from build123d import *

# Parameters (mm, degrees)
SKETCH1_R           = 1.5
SKETCH1_R_2         = 1
SKETCH1_W           = 2
SKETCH1_H           = 7
BOSS_EXTRUDE1_DEPTH = 5


with BuildPart() as part:
    # Sketch1 → Boss-Extrude1 (new body)
    with BuildSketch(Plane.XY):
        with BuildLine():
            Line((10.74521866, -60), (-20.072092256, -60))
            ThreePointArc((-20.072092256, -60), (-4.663436798, -26.922179377), (10.74521866, -60))
        make_face()
        with Locations((7.518690065, -56.019210774)):
            Circle(SKETCH1_R, mode=Mode.SUBTRACT)
        with Locations((-18.522064611, -53.115425948)):
            Circle(SKETCH1_R, mode=Mode.SUBTRACT)
        with Locations((-2.986935847, -32.015363278)):
            Circle(SKETCH1_R, mode=Mode.SUBTRACT)
        with Locations((1.346970842, -41.03959236)):
            Circle(SKETCH1_R_2, mode=Mode.SUBTRACT)
        with Locations((1.346970842, -53.06040764)):
            Circle(SKETCH1_R_2, mode=Mode.SUBTRACT)
        with Locations((-10.673844438, -53.06040764)):
            Circle(SKETCH1_R_2, mode=Mode.SUBTRACT)
        with Locations((-10.673844438, -41.03959236)):
            Circle(SKETCH1_R_2, mode=Mode.SUBTRACT)
        with Locations((-0.163436798, -47.05)):
            Rectangle(SKETCH1_W, SKETCH1_H, mode=Mode.SUBTRACT)
    extrude(amount=BOSS_EXTRUDE1_DEPTH)


solid = part.part
Build history of the part. All positions in model axes, mm. A direction names the side the tool comes from. Round coordinates to 2 decimals unless told otherwise and drop trailing zeros. Write each loop counter-clockwise with the first axis right and the second up, starting at its lowest first coordinate (ties: lowest second). Pieces come first, ordered by that corner, then holes. Notation, with made-up numbers: M -13,69.5 L 12,69.5 A23 cw 12,88.5 Z; hole C 75,56 d5. An arc over 180 degrees is marked long. Use CSV: the item, a comma, the result in double quotes.
1. Saw through at A-A (y = -47.05). Give the cut face in (x, z).
Reply:
outline,"M -24.79,0 L -1.16,0 L -1.16,5 L -24.79,5 Z; M 0.84,0 L 15.46,0 L 15.46,5 L 0.84,5 Z"
2. Wall check: probe 1 along X at (y, z) = (-53, 4.2); probe 2 along Y at (x, z) = (-11, 2.6); probe 3 along Y at (x, z) = (-10.5, 3.95). Give the ranges that are in metal, low to high. Write a range as from..to.
Reply:
probe 1,"x = -23.89..-20.02, -17.03..-11.67, -9.68..0.35, 2.35..14.56"
probe 2,"y = -60..-54.01, -52.12..-41.98, -40.09..-27.95"
probe 3,"y = -60..-54.05, -52.08..-42.02, -40.05..-27.79"
3. Saw through at D-D (x = 10). Give the cut face in (y, z), plus the area to 3 significant figures.
Reply:
outline,"M -60,0 L -33.26,0 L -33.26,5 L -60,5 Z"
area,"134 mm²"
4. Saw through at B-B (x = -3). Give the cut face in (y, z).
Reply:
outline,"M -60,0 L -33.52,0 L -33.52,5 L -60,5 Z; M -30.52,0 L -26.99,0 L -26.99,5 L -30.52,5 Z"
5. Two-plate mould, pull along Y, no slides. Class faces 1 (the face through (-4, -60, 2)), 2 (the face through (1.13, -42.016, 2.465)), 3 (the face through (0.837, -47, 2)), 4 (the face through (-4, -43, 0)): +Y half, -Y half, draft (parallel to the pull), parting line (faces both ways), or undercut.
Reply:
face 1,"-Y half"
face 2,"undercut"
face 3,"undercut"
face 4,"draft"
6. Tool access for faces 5 (the face through (0, -43.55, 2)), 6 (the face through (-4, -43, 5)): list every direction of +Z, -Z, +X, -X, +Y, -Y with a clear straight run to the whole face (end or side of a thin tool).
Reply:
face 5,"+Z, -Z"
face 6,"+Z, +X, -X, +Y, -Y"
7. Saw through at C-C (z = 3.6). State how many separate pieces and enclosed holes the cut face has, plus the area to 3 significant figures.
Reply:
separate pieces,"1"
enclosed holes,"8"
area,"1,070 mm²"
8. Flat gauge pins, fed straight in: pin 1 (1.5 mm diameter, centred on y = -48.5, z = 3.5, fed in from -X); pin 2 (2 mm diameter, centred on x = 0.5, z = 3.5, fed in from +Y). Where does each tip first touch, or does it go through?
Reply:
pin 1,"stops at x = -24.78"
pin 2,"stops at y = -27.36"
